Could you check a few things on this model? Use its own coordinates, in mm. Face numbers are marked on the shaded views. A direction names the side the tool comes from. Give positions to 0.01 mm unless a question says otherwise; leave off trailing zeros. Write each loop counter-clockwise with the first axis right and the second up, starting at its lowest first coordinate (ties: lowest second). Pieces come first, ordered by that corner, then holes. Notation, with made-up numbers: M 28,-31 L 76,-31 A31 cw 76,-7 Z; hole C -21.5,78.25 d3. An arc over 180 degrees is marked long. One line per item, written item: value.
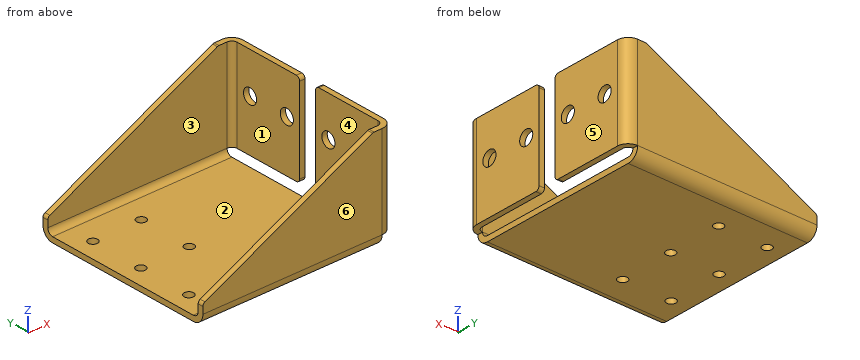
Autodesk Inventor part; units mm, degrees
ref_plane "YZ Plane" through (0, 0, 0) normal (1, 0, 0) x (0, 1, 0)
ref_plane "XZ Plane" through (0, 0, 0) normal (0, 1, 0) x (-1, 0, 0)
ref_plane "XY Plane" through (0, 0, 0) normal (0, 0, 1) x (1, 0, 0)
sketch "スケッチ1" plane through (0, 0, 0) normal (0, 0, 1) x (1, 0, 0)
  line L0 (-50, -50) -> (50, -50)
  line L1 (50, -50) -> (50, 50)
  line L2 (50, 50) -> (-50, 50)
  line L3 (-50, 50) -> (-50, -50)
  line L4 (-50, -50) -> (50, 50) construction
  line L5 (50, -50) -> (-50, 50) construction
  point P0 (0, 0)
  dimension "d0" = 100
  dimension "d1" = 100
extrude "プレート1" add sketch "スケッチ1" along normal blind 3
sketch "スケッチ2" plane through (-50, 47, 0) normal (0, 1, 0) x (-1, 0, 0)
  line L0 (-100, 0) -> (0, 0)
  line L1 (0, 0) -> (0, 57)
  line L2 (0, 57) -> (-100, 57)
  line L3 (-100, 57) -> (-100, 0)
edge flange "フランジ1" height 57 angle 90 thickness 3 bend radius 3 thickness toward (0, 1, 0) relief tear relief width 3 relief depth 1.5 corner gap 3 corner form 0 edges at (0, 50, 3) (0, -50, 3) wall of the first edge with corners at (50, 47, 0) (-50, 47, 0) (-50, 47, 57) (50, 47, 57)
bend "曲げ1"
corner "コーナー1"
sketch "スケッチ3" plane through (53, 44, 57) normal (1, 0, 0) x (0, 1, 0)
  line L0 (0, -51) -> (0, 0)
  line L1 (0, 0) -> (-39, 0)
  line L2 (-39, 0) -> (-39, -51)
  line L3 (-39, -51) -> (0, -51)
edge flange "フランジ2" height 45 angle 90 thickness 3 bend radius 3 thickness toward (1, 0, 0) relief tear relief width 3 relief depth 1.5 corner gap 3 corner form 0 edges at (50, 47, 31.5) (50, -47, 31.5) wall of the first edge with corners at (53, 44, 6) (53, 44, 57) (53, 5, 57) (53, 5, 6)
bend "曲げ2"
corner "コーナー2"
sketch "スケッチ4" plane through (-50, -50, 6) normal (0, -1, 0) x (1, 0, 0)
  line L0 (0, 0) -> (0, 51)
  line L1 (0, 5) -> (95, 51)
  line L2 (0, 51) -> (100, 51)
  line L3 (0, 0) -> (100, 0)
  line L4 (100, 51) -> (100, 0)
  point P0 (50, -6)
  dimension "d23" = 5
  dimension "d24" = 5
extrude "押し出し1" cut sketch "スケッチ4" against normal through all contours L0 L2 L1
fillet "フィレット1" radius 2 8 edges at (-50, 48.5, 11) (-50, -48.5, 11) (45, 48.5, 57) (45, -48.5, 57) (54.5, 5, 57) (54.5, -5, 6) (54.5, 5, 6) (54.5, -5, 57)
sketch "スケッチ5" plane through (0, 0, 3) normal (0, 0, 1) x (1, 0, 0)
  line L0 (-40, -30) -> (-13, -30)
  line L1 (-13, -30) -> (-13, 30)
  line L2 (-13, 30) -> (-40, 30)
  line L3 (-40, 30) -> (-40, -30)
  line L4 (-40, -30) -> (-13, 30) construction
  line L5 (-13, -30) -> (-40, 30) construction
  line L6 (-50, -44) -> (-50, 44)
  point P0 (0, 0)
  point P1 (-26.5, 0)
  point P2 (-26.5, 0)
  point P3 (-40, 0)
  point P4 (-13, 0)
  dimension "d28" = 27
  dimension "d29" = 10
  dimension "d30" = 60
hole "穴1" at (-40, 0, 3) at (-13, 0, 3) at (-40, -30, 3) at (-40, 30, 3) at (-13, -30, 3) at (-13, 30, 3) direction (0, 0, -1) diameter 5.2 end through all
sketch "スケッチ6" plane through (53, 44, 6) normal (-1, 0, 0) x (0, 0, 1)
  arc A0 (0, -37) -> (2, -39) centre (2, -37) ccw
  line L0 (2, -39) -> (49, -39)
  arc A1 (49, -39) -> (51, -37) centre (49, -37) ccw
  line L1 (51, -37) -> (51, 0)
  line L2 (51, 0) -> (0, 0)
  line L3 (0, -37) -> (0, 0)
  arc A2 (2, -49) -> (0, -51) centre (2, -51) ccw
  line L4 (0, -51) -> (0, -88)
  line L5 (0, -88) -> (51, -88)
  line L6 (51, -51) -> (51, -88)
  arc A3 (51, -51) -> (49, -49) centre (49, -51) ccw
  line L7 (49, -49) -> (2, -49)
  point P0 (-6, -44)
  point P1 (28.5, -8)
  point P2 (28.5, -31)
  point P3 (28.5, -57)
  point P4 (28.5, -80)
  dimension "d38" = 22.5
  dimension "d39" = 8
  dimension "d40" = 8
  dimension "d41" = 8
  dimension "d42" = 8
hole "穴2" at (53, 36, 34.5) at (53, 13, 34.5) at (53, -13, 34.5) at (53, -36, 34.5) direction (1, 0, 0) diameter 8.2 end through all
equation "\"d36\" = Thickness"
equation "\"d48\" = Thickness"
equation "\"d2\" = Thickness"
equation "\"d3\" = BendReliefWidth"
equation "\"d4\" = BendReliefDepth"
equation "\"d5\" = MinimumRemnant"
equation "\"d6\" = TransitionRadius"
equation "\"d9\" = BendRadius"
equation "\"d10\" = CornerReliefSize"
equation "\"d11\" = GapSize"
equation "\"d12\" = JacobiRadiusSize"
equation "\"d13\" = BendReliefWidth"
equation "\"d14\" = BendReliefDepth"
equation "\"d15\" = MinimumRemnant"
equation "\"d16\" = TransitionRadius"
equation "\"d19\" = BendRadius"
equation "\"d20\" = CornerReliefSize"
equation "\"d21\" = GapSize"
equation "\"d22\" = JacobiRadiusSize"
equation "\"BendRadius\" = Thickness"
equation "\"BendReliefWidth\" = Thickness"
equation "\"BendReliefDepth\" = 0.5 * Thickness"
equation "\"CornerReliefSize\" = 4 * Thickness"
equation "\"MinimumRemnant\" = 2 * Thickness"
equation "\"TransitionRadius\" = BendRadius"
equation "\"JacobiRadiusSize\" = BendRadius"
equation "\"GapSize\" = Thickness"
properties part number "CCM_Mount_A"
1) I'm going to push flat-ended pins straight in: pin 1 (1 mm diameter, centred on y = -37, z = 24, fed in from -X); pin 2 (2.5 mm diameter, centred on x = 54, z = 25, fed in from -Y); pin 3 (2.5 mm diameter, centred on x = 55, z = 20, fed in from +Y); pin 4 (6.5 mm diameter, centred on y = -36, z = 34.5, fed in from +X). Where does each tip first touch, or does it pass through?
Outcome:
pin 1: stops at x = 53
pin 2: stops at y = -49.33
pin 3: stops at y = 48.68
pin 4: passes through
2) If we section it at B-B, the plane y = -30: Write out the boundary of the cut face in (x, z).
Outcome:
outline: M -50,0 L -42.6,0 L -42.6,3 L -50,3 Z; M -37.4,0 L -15.6,0 L -15.6,3 L -37.4,3 Z; M -10.4,0 L 50,0 L 50,3 L -10.4,3 Z; M 53,6 L 56,6 L 56,57 L 53,57 Z
3) On a 3-axis mill with a long thin cutter (end or side, diameter ignored), from which of +Z, -Z, +X, -X, +Y, -Y can I reach the whole of each face in a straight line? I mean the marked faces 1, 2 and 3. Say none if no direction works.
Outcome:
face 1: +Z, -Z, -X
face 2: +Z, +X, -X
face 3: +Z, -X
4) We'd pull the mould along Y, two halves only. Please class the marked faces 4, 5 and 6: pulls with the +Y half, pulls with the -Y half, needs draft (parallel to the pull), parting line crosses it, or undercut.
Outcome:
face 4: undercut
face 5: needs draft
face 6: pulls with the -Y half
5) If we section it at D-D, the plane x = 47: Write out the boundary of the cut face in (y, z).
Outcome:
outline: M -50,6 A6 ccw -44,0 L 44,0 A6 ccw 50,6 L 50,57 L 47,57 L 47,6 A3 cw 44,3 L -44,3 A3 cw -47,6 L -47,57 L -50,57 Z
6) Please list where these lines run through material, in increasing order: L1, parallel to X at y = 30, z = 2.25; L2, parallel to Y at x = 15, z = 9; L3, parallel to Z at x = 45.5, y = 14. Write a range as from..to.
Outcome:
L1: x = -50..-42.6, -37.4..-15.6, -10.4..50
L2: y = -50..-47, 47..50
L3: z = 0..3
7) If we section it at C-C, the plane z = 41: Write out the boundary of the cut face in (x, y).
Outcome:
outline: M 11.96,-50 L 50,-50 A6 ccw 56,-44 L 56,-5 L 53,-5 L 53,-44 A3 cw 50,-47 L 11.96,-47 Z; M 11.96,47 L 50,47 A3 cw 53,44 L 53,5 L 56,5 L 56,44 A6 ccw 50,50 L 11.96,50 Z
8) If we section it at A-A, the plane y = 0: Write out the boundary of the cut face in (x, z), then the cut area to 3 significant figures.
Outcome:
outline: M -50,0 L -42.6,0 L -42.6,3 L -50,3 Z; M -37.4,0 L -15.6,0 L -15.6,3 L -37.4,3 Z; M -10.4,0 L 50,0 L 50,3 L -10.4,3 Z
area: 269 mm^2
